Build history of the part. All positions in model axes, mm. A direction names the side the tool comes from. Round coordinates to 2 decimals unless told otherwise and drop trailing zeros. Loops run counter-clockwise (first coordinate to the right, second up) from the corner with the lowest first, then second, coordinate; pieces in that order, holes last. Notation, with made-up numbers: (2.25, 25.25) - (56.25, 25.25) arc R29 cw to (56.25, 49.25) - close; hole circle Ø9 at (-30, 86). An arc over 180 degrees is marked (long way). Use a Markdown table: item, result.
from build123d import *

# Parameters (mm, degrees)
SKETCH1_W                     = 103.632
SKETCH1_H                     = 105.664
BOSS_EXTRUDE1_DEPTH           = 9.525
SKETCH2_W                     = 99.822
SKETCH2_H                     = 101.854
BOSS_EXTRUDE2_DEPTH           = 234.95
SKETCH4_W                     = 103.632
SKETCH4_H                     = 105.664
BOSS_EXTRUDE5_DEPTH           = 9.525
TAP_DRILL_FOR_6_32_TAP1_D     = 2.7051
TAP_DRILL_FOR_6_32_TAP1_DEPTH = 3.97002
TAP_DRILL_FOR_6_32_TAP1_TIP   = 0.81269403


with BuildPart() as part:
    # Sketch1 → Boss-Extrude1 (new body)
    with BuildSketch(Plane.XY):
        with Locations((51.816, -52.832)):
            Rectangle(SKETCH1_W, SKETCH1_H)
    extrude(amount=-BOSS_EXTRUDE1_DEPTH)

    # Sketch2 → Boss-Extrude2 (add)
    with BuildSketch(Plane(origin=(0, 0, -9.525), x_dir=(-1, 0, 0), z_dir=(0, 0, -1))):
        with Locations((-51.816, -52.832)):
            Rectangle(SKETCH2_W, SKETCH2_H)
    extrude(amount=BOSS_EXTRUDE2_DEPTH)

    # Sketch4 → Boss-Extrude5 (add)
    with BuildSketch(Plane(origin=(0, 0, -244.475), x_dir=(-1, 0, 0), z_dir=(0, 0, -1))):
        with Locations((-51.816, -52.832)):
            Rectangle(SKETCH4_W, SKETCH4_H)
    extrude(amount=BOSS_EXTRUDE5_DEPTH)

    # Tap Drill for #6-32 Tap1
    with Locations(Plane(origin=(0, -103.759, 0), x_dir=(-1, 0, 0), z_dir=(0, -1, 0))):
        with Locations((-88.3285, 234.95), (-15.3035, 234.95), (-88.3285, 19.05), (-15.3035, 19.05)):
            Hole(TAP_DRILL_FOR_6_32_TAP1_D / 2, depth=TAP_DRILL_FOR_6_32_TAP1_DEPTH)
            with Locations((0, 0, -(TAP_DRILL_FOR_6_32_TAP1_DEPTH + TAP_DRILL_FOR_6_32_TAP1_TIP / 2))):  # 118° drill point
                Cone(0, TAP_DRILL_FOR_6_32_TAP1_D / 2, TAP_DRILL_FOR_6_32_TAP1_TIP, mode=Mode.SUBTRACT)


solid = part.part
Q1. Which spindle directions (+Z, -Z, +X, -X, +Y, -Y) get a long thin tool onto all of the face, cutting with end or side? Do faces 1 (the face through (1.905, -54, -125)), 2 (the face through (101.727, -54, -125)), 3 (the face through (53, -1.905, -125)). Say none if no direction does.
Results found:
| item | result |
|---|---|
| face 1 | -X, +Y, -Y |
| face 2 | +X, +Y, -Y |
| face 3 | +X, -X, +Y |
Q2. Cut at C-C, the plane z = -206.5. List the corners of the cut face in (x, y) (3 decimals), plus the area to 3 significant figures.
Results found:
| item | result |
|---|---|
| outline | (1.905, -103.759) - (101.727, -103.759) - (101.727, -1.905) - (1.905, -1.905) - close |
| area | 10,200 mm2 |
Q3. Cut at B-B, the plane x = 8. List the corners of the cut face in (y, z) (3 decimals).
Results found:
| item | result |
|---|---|
| outline | (-105.664, -254) - (0, -254) - (0, -244.475) - (-1.905, -244.475) - (-1.905, -9.525) - (0, -9.525) - (0, 0) - (-105.664, 0) - (-105.664, -9.525) - (-103.759, -9.525) - (-103.759, -244.475) - (-105.664, -244.475) - close |
Q4. Cut at A-A, the plane y = -44. List the corners of the cut face in (x, z) (3 decimals).
Results found:
| item | result |
|---|---|
| outline | (0, -254) - (103.632, -254) - (103.632, -244.475) - (101.727, -244.475) - (101.727, -9.525) - (103.632, -9.525) - (103.632, 0) - (0, 0) - (0, -9.525) - (1.905, -9.525) - (1.905, -244.475) - (0, -244.475) - close |
Q5. Drop flat-ended pins along their axis: pin 1 (3.5 mm diameter, centred on x = 88.33, z = -234.95, fed in from +Y) (3 decimals); pin 2 (1 mm diameter, centred on x = 81, z = -98, fed in from -Y); pin 3 (4 mm diameter, centred on x = 43.5, y = -16.5, fed in from +Z); pin 4 (6 mm diameter, centred on y = -76, z = -106, fed in from -X) (3 decimals). Give the stop position or say it passes through.
Results found:
| item | result |
|---|---|
| pin 1 | stops at y = -1.905 |
| pin 2 | stops at y = -103.76 |
| pin 3 | stops at z = 0 |
| pin 4 | stops at x = 1.905 |
Q6. Probe line 1 (X direction, y = -101.45, z = -19.05) (3 decimals); line 2 (X direction, y = -77.5, z = -89) (3 decimals); line 3 (Y direction, x = 6, z = -62) (3 decimals). List the from-to ranges inside material, lowest first.
Results found:
| item | result |
|---|---|
| line 1 | x = 1.905 to 13.951, 16.656 to 86.976, 89.681 to 101.727 |
| line 2 | x = 1.905 to 101.727 |
| line 3 | y = -103.759 to -1.905 |
